```python
from build123d import *

# Parameters (mm, degrees)
SKETCH1_R           = 3.05
SKETCH1_R_2         = 1.55
BOSS_EXTRUDE1_DEPTH = 2
SKETCH3_R           = 3.05
BOSS_EXTRUDE2_DEPTH = 2
FILLET1_R           = 2


with BuildPart() as part:
    # Sketch1 → Boss-Extrude1 (new body)
    with BuildSketch(Plane(origin=(0, 0, 0), x_dir=(1, 0, 0), z_dir=(0, 1, 0))):
        Circle(SKETCH1_R)
        Circle(SKETCH1_R_2, mode=Mode.SUBTRACT)
    extrude(amount=BOSS_EXTRUDE1_DEPTH)

    # Sketch3 → Boss-Extrude2 (add)
    with BuildSketch(Plane(origin=(0, 2, 0), x_dir=(1, 0, 0), z_dir=(0, 1, 0))):
        Circle(SKETCH3_R)
    extrude(amount=BOSS_EXTRUDE2_DEPTH)

    # Fillet1
    fillet1_edges = [part.edges().sort_by_distance(p)[0] for p in [
        (-3.05, 4, 0),
    ]]
    fillet(fillet1_edges, radius=FILLET1_R)


solid = part.part
```
For this review, take the finished solid that the model builds, in its own axes (mm). A direction names the side the tool comes from. Give positions to 0.01 mm unless a question says otherwise; leave off trailing zeros. Loops run counter-clockwise (first coordinate to the right, second up) from the corner with the lowest first, then second, coordinate; pieces in that order, holes last. Notation, with made-up numbers: M 77.25,28 L 104.25,28 A15 cw 104.25,39 Z; hole C 18,13.5 d1. An arc over 180 degrees is marked long. One line per item, written item: value. Start each with the question number.
Q1. For L1, parallel to Z at x = 0, y = 1.8; L2, parallel to Y at x = 0.5, z = -0.5, list the stretches that pass through material, from the lowest coordinate up.
Q2. Add section A-A (y = 0.35). Give the boundary of the cut face in (x, z), and give its area (3 significant figures).
Q3. Draft analysis for pull direction Z (two halves, no side actions). For faces 1 (the face through (-3.047, 0.986, -0.134)), 2 (the face through (0.715, 0.986, 1.375)), 3 (the face through (0, 4, 0)), state which applies: released by +Z, released by -Z, zero draft, split by the parting line, or undercut.
Q4. Machinability: for faces 4 (the face through (0, 2, 0)), 5 (the face through (1.3, 0, 1.3)), which of the approach directions +Z, -Z, +X, -X, +Y, -Y give a long, thin tool a straight path to every point of the face, cutting with its end or side? Answer none if there is none.
Reply:
1. L1: -3.05 to -1.55, 1.55 to 3.05
1. L2: 2 to 4
2. outline: C 0,0 d6.1; hole C 0,0 d3.1
2. area: 21.7 mm²
3. face 1: split by the parting line
3. face 2: undercut
3. face 3: zero draft
4. face 4: -Y
4. face 5: +Z, -Z, +X, -X, -Y
